Design review of the part built by this model. Coordinates are the model's own, in mm. Face numbers are marked on the shaded views. A direction names the side the tool comes from. Round coordinates to 2 decimals unless told otherwise and drop trailing zeros. Loops run counter-clockwise (first coordinate to the right, second up) from the corner with the lowest first, then second, coordinate; pieces in that order, holes last. Notation, with made-up numbers: (-17, 28) - (11, 28) arc R11 cw to (11, 40) - close; hole circle Ø7 at (35, 23.25). An arc over 180 degrees is marked (long way). Use one line per item in the form item = value. Start each with the question number.
(1) Machinability: for the marked faces 4, 5 and 6, which of the approach directions +Z, -Z, +X, -X, +Y, -Y give a long, thin tool a straight path to every point of the face, cutting with its end or side? Answer none if there is none.
(2) Wall thickness on probe 1 along Z at (x, y) = (-2.5, 4.75); probe 2 along X at (y, z) = (-1.5, 2); probe 3 along Y at (x, z) = (1.75, -1): over which ranges is each line inside the solid? List them lowest first. Write a range as [from, to].
(3) For pin 1 (1.7 mm diameter, centred on x = -1.5, z = -1, fed in from +Y); pin 2 (5.5 mm diameter, centred on x = 1, z = -0.5, fed in from -Y); pin 3 (0.6 mm diameter, centred on y = 6.5, z = -11.5, fed in from -X), all flat-tipped, find the tip position at first contact; note any pin that passes through.
(4) We need section A-A, the plane y = 2.75. Write out the cut boundary in (x, z).
(5) We need section D-D, the plane x = -5.5. Write out the cut boundary in (y, z), then the cut area to 3 significant figures.
(6) We need section B-B, the plane x = -1.25. Write out the cut boundary in (y, z).
(7) The part is to be moulded in two halves that separate along Y. For the marked faces 1, 2 and 3, say which applies: released by +Y, released by -Y, zero draft, split by the parting line, or undercut.
(8) We need section C-C, the plane z = -6. Write out the cut boundary in (x, y).
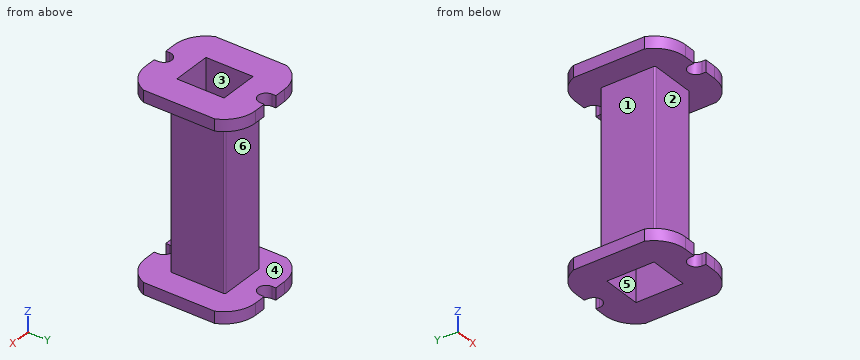
from build123d import *

# Parameters (mm, degrees)
SKETCH_1_W               = 6
SKETCH_1_H               = 7
SKETCH_1_W_2             = 5
SKETCH_1_H_2             = 6
EXTRUDE_1_DEPTH          = 12.5
SKETCH_2_W               = 6
SKETCH_2_H               = 7
EXTRUDE_2_DEPTH          = 1.5
SKETCH_3_R               = 19.100398606
SKETCH_3_W               = 18.715870292
SKETCH_3_H               = 14
CUT_EXTRUDE_1_DEPTH      = 28.522717889
CUT_EXTRUDE_2_DEPTH      = 27.762847382
CUT_EXTRUDE_3_DEPTH      = 27.762847382
CUT_EXTRUDE_3_DEPTH_BACK = 27.762847382
FILLET_1_R               = 0.2


with BuildPart() as part:
    # 草图1 → 凸台-拉伸1 (new, symmetric)
    with BuildSketch(Plane.XY):
        Rectangle(SKETCH_1_W, SKETCH_1_H)
        Rectangle(SKETCH_1_W_2, SKETCH_1_H_2, mode=Mode.SUBTRACT)
    extrude(amount=EXTRUDE_1_DEPTH, both=True)

    # 草图2 → 凸台-拉伸2 (add)
    with BuildSketch(Plane.XY.offset(12.5)):
        with BuildLine():
            Line((-6.5, 6.92820323), (-6.5, -6.92820323))
            ThreePointArc((-6.5, -6.92820323), (0, -9.5), (6.5, -6.92820323))
            Line((6.5, -6.92820323), (6.5, 6.92820323))
            ThreePointArc((6.5, 6.92820323), (0, 9.5), (-6.5, 6.92820323))
        make_face()
        Rectangle(SKETCH_2_W, SKETCH_2_H, mode=Mode.SUBTRACT)
    extrude_2 = extrude(amount=-EXTRUDE_2_DEPTH)

    # 镜向1: 凸台-拉伸2 across plane
    add(extrude_2.mirror(Plane.XY))

    # 草图3 → 切除-拉伸1 (cut, through all)
    with BuildSketch(Plane.XY.offset(12.5)):
        Circle(SKETCH_3_R)
        Rectangle(SKETCH_3_W, SKETCH_3_H, mode=Mode.SUBTRACT)
    extrude(amount=-CUT_EXTRUDE_1_DEPTH, mode=Mode.SUBTRACT)

    # 草图4 → 切除-拉伸2 (cut, through all)
    with BuildSketch(Plane.XY.offset(12.5)):
        with BuildLine():
            Line((-6.5, 6.92820323), (-6.5, 3))
            ThreePointArc((-6.5, 3), (-5.328427125, 5.828427125), (-2.5, 7))
            Line((-2.5, 7), (-6.422616289, 7))
            ThreePointArc((-6.422616289, 7), (-6.461407868, 6.964209098), (-6.5, 6.92820323))
        make_face()
        with BuildLine():
            ThreePointArc((2.5, 7), (5.328427125, 5.828427125), (6.5, 3))
            Line((6.5, 3), (6.5, 6.92820323))
            ThreePointArc((6.5, 6.92820323), (6.461407868, 6.964209098), (6.422616289, 7))
            Line((6.422616289, 7), (2.5, 7))
        make_face()
        with BuildLine():
            ThreePointArc((6.5, -3), (5.328427127, -5.828427123), (2.500000005, -7))
            Line((2.500000005, -7), (6.422616289, -7))
            ThreePointArc((6.422616289, -7), (6.461407868, -6.964209098), (6.5, -6.92820323))
            Line((6.5, -6.92820323), (6.5, -3))
        make_face()
        with BuildLine():
            ThreePointArc((-6.5, -6.92820323), (-6.461407868, -6.964209098), (-6.422616289, -7))
            Line((-6.422616289, -7), (-2.499999995, -7))
            ThreePointArc((-2.499999995, -7), (-5.328427123, -5.828427127), (-6.5, -3))
            Line((-6.5, -3), (-6.5, -6.92820323))
        make_face()
    extrude(amount=-CUT_EXTRUDE_2_DEPTH, mode=Mode.SUBTRACT)

    # 草图5 → 切除-拉伸3 (cut, two sides: drawn at the far end of the back side and taken through both)
    with BuildSketch(Plane.XY.offset(12.5).offset(-CUT_EXTRUDE_3_DEPTH_BACK)):
        with BuildLine():
            Line((1, 7), (-1, 7))
            Line((-1, 7), (-1, 6.5))
            ThreePointArc((-1, 6.5), (0, 5.5), (1, 6.5))
            Line((1, 6.5), (1, 7))
        make_face()
        with BuildLine():
            Line((-1, -6.5), (-1, -7))
            Line((-1, -7), (1, -7))
            Line((1, -7), (1, -6.5))
            ThreePointArc((1, -6.5), (0, -5.5), (-1, -6.5))
        make_face()
        with BuildLine():
            Line((-6.2, -4.519868415), (-6.2, 4.519868415))
            ThreePointArc((-6.2, 4.519868415), (-6.424283374, 3.774596669), (-6.5, 3))
            Line((-6.5, 3), (-6.5, -3))
            ThreePointArc((-6.5, -3), (-6.424283374, -3.774596669), (-6.2, -4.519868415))
        make_face()
        with BuildLine():
            ThreePointArc((6.5, 3), (6.424283374, 3.774596669), (6.2, 4.519868415))
            Line((6.2, 4.519868415), (6.2, -4.519868415))
            ThreePointArc((6.2, -4.519868415), (6.424283374, -3.774596669), (6.5, -3))
            Line((6.5, -3), (6.5, 3))
        make_face()
    extrude(amount=CUT_EXTRUDE_3_DEPTH + CUT_EXTRUDE_3_DEPTH_BACK, mode=Mode.SUBTRACT)

    # 圆角1
    fillet_1_edges = [part.edges().sort_by_distance(p)[0] for p in [
        (-3, 3.5, 0),
        (3, 3.5, 0),
        (3, -3.5, 0),
        (-3, -3.5, 0),
    ]]
    fillet(fillet_1_edges, radius=FILLET_1_R)


solid = part.part
Data:
q1.face_4 = none
q1.face_5 = +Z, -Z
q1.face_6 = +X, -X, +Y
q2.probe_1 = [-12.5, -11], [11, 12.5]
q2.probe_2 = [-3, -2.5], [2.5, 3]
q2.probe_3 = [-3.5, -3], [3, 3.5]
q3.pin_1 = 3.5
q3.pin_2 = -3.5
q3.pin_3 = -4.9
q4.outline = (-6.2, -12.5) - (-2.5, -12.5) - (-2.5, 12.5) - (-6.2, 12.5) - (-6.2, 11) - (-3, 11) - (-3, -11) - (-6.2, -11) - close; (2.5, -12.5) - (6.2, -12.5) - (6.2, -11) - (3, -11) - (3, 11) - (6.2, 11) - (6.2, 12.5) - (2.5, 12.5) - close
q5.outline = (-5.65, -12.5) - (5.65, -12.5) - (5.65, -11) - (-5.65, -11) - close; (-5.65, 11) - (5.65, 11) - (5.65, 12.5) - (-5.65, 12.5) - close
q5.area = 33.9 mm^2
q6.outline = (-7, -12.5) - (-3, -12.5) - (-3, 12.5) - (-7, 12.5) - (-7, 11) - (-3.5, 11) - (-3.5, -11) - (-7, -11) - close; (3, -12.5) - (7, -12.5) - (7, -11) - (3.5, -11) - (3.5, 11) - (7, 11) - (7, 12.5) - (3, 12.5) - close
q7.face_1 = zero draft
q7.face_2 = released by -Y
q7.face_3 = undercut
q8.outline = (-3, -3.3) arc R0.2 ccw to (-2.8, -3.5) - (2.8, -3.5) arc R0.2 ccw to (3, -3.3) - (3, 3.3) arc R0.2 ccw to (2.8, 3.5) - (-2.8, 3.5) arc R0.2 ccw to (-3, 3.3) - close; hole (-2.5, -3) - (2.5, -3) - (2.5, 3) - (-2.5, 3) - close
